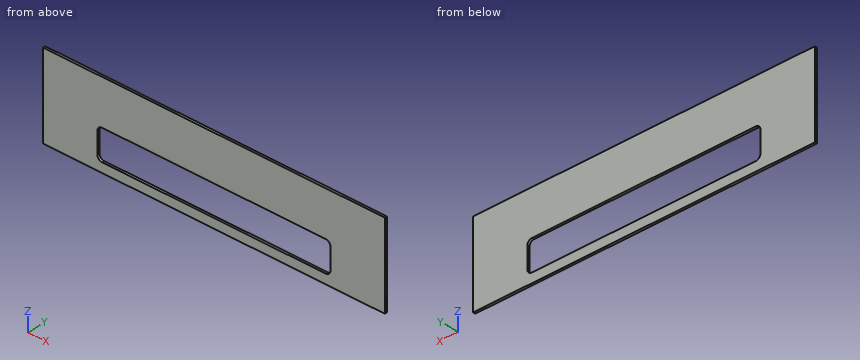
from build123d import *

# Parameters (mm, degrees)
SKETCH1_W           = 232.41
SKETCH1_H           = 57.15
BOSS_EXTRUDE1_DEPTH = 1.5875
SKETCH2_W           = 158.496
SKETCH2_H           = 20.574
CUT_EXTRUDE1_DEPTH  = 2.5875
FILLET1_R           = 3.175


with BuildPart() as part:
    # Sketch1 → Boss-Extrude1 (new body)
    with BuildSketch(Plane(origin=(0, 0, 0), x_dir=(1, 0, 0), z_dir=(0, 1, 0))):
        Rectangle(SKETCH1_W, SKETCH1_H)
    extrude(amount=BOSS_EXTRUDE1_DEPTH)

    # Sketch2 → Cut-Extrude1 (cut, through all)
    with BuildSketch(Plane(origin=(0, 1.5875, 0), x_dir=(1, 0, 0), z_dir=(0, 1, 0))):
        with Locations((0, 11.938)):
            Rectangle(SKETCH2_W, SKETCH2_H)
    extrude(amount=-CUT_EXTRUDE1_DEPTH, mode=Mode.SUBTRACT)

    # Fillet1
    fillet1_edges = [part.edges().sort_by_distance(p)[0] for p in [
        (-79.248, 0.79375, -1.651),
        (-79.248, 0.79375, -22.225),
        (79.248, 0.79375, -22.225),
        (79.248, 0.79375, -1.651),
    ]]
    fillet(fillet1_edges, radius=FILLET1_R)


solid = part.part
Geometry: final body of the model. Coordinates: model frame, mm. Coordinates: 2 decimals unless noted, no trailing zeros. Order: outer loops, then holes, each group sorted by start corner. A loop starts at its lowest first (then second) coordinate and runs counter-clockwise, first axis right, second up.
1) Section B-B (x = 1). Return loops of the section in (y, z) (1 decimal), then the cut area to 3 significant figures.
Result sheet:
outline: (0, -28.6) - (1.6, -28.6) - (1.6, -22.2) - (0, -22.2) - close; (0, -1.7) - (1.6, -1.7) - (1.6, 28.6) - (0, 28.6) - close
area: 58.1 mm2
2) Ray query, probe 1 along Z at (x, y) = (-56, 1.45) (3 decimals); probe 2 along X at (y, z) = (0.9, -7.5) (3 decimals). Return the intervals inside material, ascending.
Result sheet:
probe 1: z = -28.575 to -22.225, -1.651 to 28.575
probe 2: x = -116.205 to -79.248, 79.248 to 116.205
3) Section A-A (z = -14). Return loops of the section in (x, y) (1 decimal), then the cut area to 3 significant figures.
Result sheet:
outline: (-116.2, 0) - (-79.2, 0) - (-79.2, 1.6) - (-116.2, 1.6) - close; (79.2, 0) - (116.2, 0) - (116.2, 1.6) - (79.2, 1.6) - close
area: 117 mm2
4) Section C-C (y = 1.25). Return loops of the section in (x, z) (3 decimals), then the cut area to 3 significant figures.
Result sheet:
outline: (-116.205, -28.575) - (116.205, -28.575) - (116.205, 28.575) - (-116.205, 28.575) - close; hole (-79.248, -19.05) arc R3.175 ccw to (-76.073, -22.225) - (76.073, -22.225) arc R3.175 ccw to (79.248, -19.05) - (79.248, -4.826) arc R3.175 ccw to (76.073, -1.651) - (-76.073, -1.651) arc R3.175 ccw to (-79.248, -4.826) - close
area: 10,000 mm2
